```python
from build123d import *

# Parameters (mm, degrees)
SWEEP1_PROFILE_R    = 2
BOSS_EXTRUDE1_DEPTH = 5
SKETCH10_R          = 1.75
CUT_EXTRUDE1_DEPTH  = 200
CUT_EXTRUDE3_REACH  = 6.012
SKETCH35_R          = 1.5


with BuildPart() as part:
    # Sweep1: sweep along a path in Sketch2
    with BuildLine(Plane(origin=(0, 0, 0), x_dir=(1, 0, 0), z_dir=(0, 1, 0))) as sweep1_path:
        Line((-100, 0), (100, 0))
    # Sweep1 profile (on start of the path) → Sweep1 (sweep)
    with BuildSketch(Plane(origin=(-100, 0, 0), x_dir=(0, 0, 1), z_dir=(1, 0, 0))):
        Circle(SWEEP1_PROFILE_R)
    sweep(path=sweep1_path.line)

    # Sketch9 → Boss-Extrude1 (add)
    with BuildSketch(Plane.ZY.offset(100)):
        Polygon((1.98826653, -1.174789146), (2.01153051, 1.134494752), (0.023263979, 2.309283898), (-1.98826653, 1.174789146), (-2.01153051, -1.134494752), (-0.023263979, -2.309283898), align=None)
    extrude(amount=BOSS_EXTRUDE1_DEPTH)

    # Sketch10 → Cut-Extrude1 (cut)
    with BuildSketch(Plane(origin=(100, 0, 0), x_dir=(0, 0, -1), z_dir=(1, 0, 0))):
        Circle(SKETCH10_R)
    extrude(amount=-CUT_EXTRUDE1_DEPTH, mode=Mode.SUBTRACT)

    # Sketch35 → Cut-Extrude3 (cut, up to next)
    with BuildSketch(Plane.XY.offset(2), mode=Mode.PRIVATE) as cut_extrude3_sk1:
        with Locations((65, 0)):
            Circle(SKETCH35_R)
    cut_extrude3_tool1 = extrude(cut_extrude3_sk1.sketch, amount=-CUT_EXTRUDE3_REACH, mode=Mode.PRIVATE) & part.part
    add(cut_extrude3_tool1.solids().sort_by_distance((65, 0, 2))[0], mode=Mode.SUBTRACT)
    # Sketch35 → Cut-Extrude3 (cut, up to next)
    with BuildSketch(Plane.XY.offset(2), mode=Mode.PRIVATE) as cut_extrude3_sk2:
        with Locations((-65, 0)):
            Circle(SKETCH35_R)
    cut_extrude3_tool2 = extrude(cut_extrude3_sk2.sketch, amount=-CUT_EXTRUDE3_REACH, mode=Mode.PRIVATE) & part.part
    add(cut_extrude3_tool2.solids().sort_by_distance((-65, 0, 2))[0], mode=Mode.SUBTRACT)


solid = part.part
```
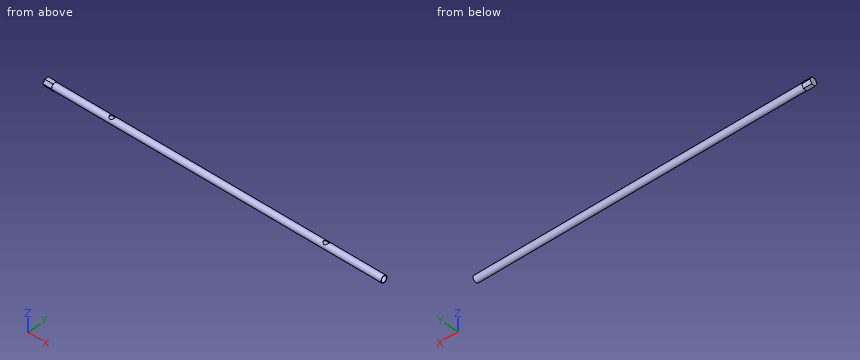
Could you check a few things on this model? Use its own coordinates, in mm. Give positions to 0.01 mm unless a question says otherwise; leave off trailing zeros. Order: outer loops, then holes, each group sorted by start corner. A loop starts at its lowest first (then second) coordinate and runs counter-clockwise, first axis right, second up.
Q1. Suppose I cut it at A-A, the plane x = 42. Write out the boundary of the cut face in (y, z).
Q2. I'm going to push flat-ended pins straight in: P1, Ø1, axis at y = -0.5, z = 0, coming from the +X side; P2, Ø1.5, axis at x = -78, y = 1, coming from the -Z side; P3, Ø1, axis at x = -8.5, y = 0.5, coming from the +Z side. Where does each tip first touch, or does it pass through?
Q3. If I drill on line 1 along Z through (x, y) = (-50, -0.3); line 2 along X through (y, z) = (0, 1.7), over which ranges is the centre line in solid material (lowest first)?
Solution:
1. outline: circle Ø4 at (0, 0); hole circle Ø3.5 at (0, 0)
2. P1: stops at x = -100
2. P2: stops at z = -1.98
2. P3: stops at z = 2
3. line 1: z = -1.98 to -1.72, 1.72 to 1.98
3. line 2: x = -105 to -100
